from build123d import *

# Parameters (mm, degrees)
SKETCH_W     = 38
SKETCH_H     = 70
PAD_DEPTH    = 8
SKETCH001_W  = 58
SKETCH001_H  = 15
PAD001_DEPTH = 9


with BuildPart() as part:
    # Sketch → Pad (new body)
    with BuildSketch(Plane.XY):
        Polygon((258, 0), (258, 5), (0, 5), (0, 0), (100, 0), (100, -85), (110, -85), (148, -85), (158, -85), (158, 0), align=None)
        with Locations((129, -35)):
            Rectangle(SKETCH_W, SKETCH_H, mode=Mode.SUBTRACT)
    extrude(amount=PAD_DEPTH)

    # Sketch001 (on Face16 of Pad) → Pad001 (join)
    with BuildSketch(Plane.XY.offset(8)):
        with Locations((129, -77.5)):
            Rectangle(SKETCH001_W, SKETCH001_H)
    extrude(amount=PAD001_DEPTH)


solid = part.part
The listing builds one solid part. Answer for the finished solid, in the listing's coordinates (mm). A direction names the side the tool comes from. Coordinates: 2 decimals unless noted, no trailing zeros. Loops run counter-clockwise (first coordinate to the right, second up) from the corner with the lowest first, then second, coordinate; pieces in that order, holes last.
1) A tool of negligible diameter and unlimited length cuts with its end or side. For faces 5 (the face through (158, -53, 5)), 6 (the face through (109, -30, 0)), 7 (the face through (110, -35, 4)), 8 (the face through (100, -53, 5)), 9 (the face through (138, 1, 8)), from which of +Z, -Z, +X, -X, +Y, -Y can it reach the whole face along a straight path? Write none if from no direction.
2) Find section A-A on y = -51. Write down the section's boundary in (x, z), then the cut area to 3 significant figures.
3) Flat-ended cylindrical pins translate along their axes: pin 1 Ø6.5 at (y, z) = (-49, 4) entering from -X; pin 2 Ø2.5 at (x, z) = (72, 2) entering from -Y; pin 3 Ø2.5 at (y, z) = (-42, 2) entering from +X. Find the tip coordinate at first contact, or state that the pin passes through.
4) Find section C-C on x = 65. Write down the section's boundary in (y, z).
5) Find the intervals of material crossed by L1, parallel to X at y = -33, z = 1.5; L2, parallel to Y at x = 236, z = 3.5; L3, parallel to Y at x = 119, z = 6.25, in increasing order.
6) Determine the mould class of faces 1 (the face through (148, -35, 4)), 2 (the face through (258, 2, 4)), 3 (the face through (129, -70, 8)), 4 (the face through (207, 0, 4)) for opening direction X: pulls with the +X half, pulls with the -X half, needs draft (parallel to the pull), parting line crosses it, or undercut.
7) Find section D-D on y = -76.5. Write down the section's boundary in (x, z).
8) Find section B-B on z = 5.5. Write down the section's boundary in (x, y), then the cut area to 3 significant figures.
Values:
1. face 5: +Z, -Z, +X, -Y
1. face 6: -Z, +X, -X, +Y, -Y
1. face 7: +Z, -Z
1. face 8: +Z, -Z, -X, -Y
1. face 9: +Z, +X, -X, +Y
2. outline: (100, 0) - (110, 0) - (110, 8) - (100, 8) - close; (148, 0) - (158, 0) - (158, 8) - (148, 8) - close
2. area: 160 mm2
3. pin 1: stops at x = 100
3. pin 2: stops at y = 0
3. pin 3: stops at x = 158
4. outline: (0, 0) - (5, 0) - (5, 8) - (0, 8) - close
5. L1: x = 100 to 110, 148 to 158
5. L2: y = 0 to 5
5. L3: y = -85 to -70, 0 to 5
6. face 1: undercut
6. face 2: pulls with the +X half
6. face 3: undercut
6. face 4: needs draft
7. outline: (100, 0) - (158, 0) - (158, 17) - (100, 17) - close
8. outline: (0, 0) - (100, 0) - (100, -85) - (158, -85) - (158, 0) - (258, 0) - (258, 5) - (0, 5) - close; hole (110, -70) - (148, -70) - (148, 0) - (110, 0) - close
8. area: 3,560 mm2
